For this review, take the finished solid that the model builds, in its own axes (mm). A direction names the side the tool comes from. Give positions to 0.01 mm unless a question says otherwise; leave off trailing zeros. Write each loop counter-clockwise with the first axis right and the second up, starting at its lowest first coordinate (ties: lowest second). Pieces come first, ordered by that corner, then holes. Notation, with made-up numbers: M 26,-33 L 36,-33 A18 ccw 36,-7 Z; hole C -3,73.25 d4. An arc over 180 degrees is marked long. Use one line per item in the form item = value. Start each with the question number.
Q1. Consider section B-B on x = 0. Write out the cut boundary in (y, z) (3 decimals), and give its area (3 significant figures).
Q2. Consider section D-D on x = -26. Write out the cut boundary in (y, z).
Q3. Clearance check with flat-ended pins moving along their axes: pin 1 Ø10 at (y, z) = (49.5, 45.5) entering from +X; pin 2 Ø10 at (y, z) = (11.5, -6) entering from +X; pin 3 Ø6 at (y, z) = (29.5, -36.5) entering from -X; pin 4 Ø1.6 at (x, z) = (-13.75, -5.41) entering from -Y. State where each tip first meets the part, or that it passes through.
Q4. Consider section A-A on y = 17. Write out the cut boundary in (x, z), and give its area (3 significant figures).
Q5. Consider section C-C on z = 0. Write out the cut boundary in (x, y) (3 decimals), and give its area (3 significant figures).
Q6. For probe 1 along Z at (x, y) = (0, 27); probe 2 along Z at (x, y) = (34, 36); probe 3 along X at (y, z) = (9, -13), list the stretches that pass through material, from the lowest coordinate up. Write a range as [from, to].
Q7. Mouldability with a two-part tool opening along Z and no side actions: class faces 1 (the cylindrical face through (41.569, 27.608, 17.235)), 2 (the cylindrical face through (26.34, 29.64, -41.32)) as released by +Z, released by -Z, zero draft, split by the parting line, or undercut.
Q8. Tool access review of faces 3 (the flat face through (38, 38, -1)), 4 (the flat face through (-15, 5, 0)), 5 (the flat face through (-26.9, 2.03, -20.31)): name each direction out of +Z, -Z, +X, -X, +Y, -Y from which nothing blocks a thin tool from reaching the whole face with its end or side.
```python
from build123d import *

# Parameters (mm, degrees)
SALIENTE_EXTRUIR2_DEPTH = 4
CROQUIS4_W              = 8
CROQUIS4_H              = 26
SALIENTE_EXTRUIR4_DEPTH = 34
CORTAR_EXTRUIR1_REACH   = 35.75
CROQUIS5_W              = 10
CROQUIS5_H              = 24
CROQUIS6_R              = 1.3
CORTAR_EXTRUIR2_DEPTH   = 7
SALIENTE_EXTRUIR5_DEPTH = 38
CROQUIS10_R             = 49
CROQUIS10_R_2           = 45
SALIENTE_EXTRUIR6_DEPTH = 56
CORTAR_EXTRUIR3_DEPTH   = 38
CROQUIS12_R             = 60.625
CROQUIS12_R_2           = 49
SALIENTE_EXTRUIR8_DEPTH = 4
CROQUIS13_R             = 3.1645
CORTAR_EXTRUIR5_DEPTH   = 14
CROQUIS14_R             = 1.3
CORTAR_EXTRUIR6_DEPTH   = 5
REDONDEO1_R             = 1


with BuildPart() as part:
    # Croquis1 → Saliente-Extruir2 (new body)
    with BuildSketch(Plane(origin=(0, 0, 0), x_dir=(1, 0, 0), z_dir=(0, 1, 0))):
        with BuildLine():
            Line((-11.25, 13.407227917), (-11.25, -12.592772083))
            Line((-11.25, -12.592772083), (-29.32452611, -34.133153509))
            ThreePointArc((-29.32452611, -34.133153509), (-44.999238647, 0.261765488), (-28.925442436, 34.47199994))
            Line((-28.925442436, 34.47199994), (-11.25, 13.407227917))
        make_face()
    extrude(amount=SALIENTE_EXTRUIR2_DEPTH)

    # Croquis4 → Saliente-Extruir4 (add)
    with BuildSketch(Plane(origin=(0, 4, 0), x_dir=(1, 0, 0), z_dir=(0, 1, 0))):
        with Locations((-15.25, 0.407227917)):
            Rectangle(CROQUIS4_W, CROQUIS4_H)
    extrude(amount=SALIENTE_EXTRUIR4_DEPTH)

    # Croquis5 → Cortar-Extruir1 (cut, up to next)
    with BuildSketch(Plane(origin=(-11.25, 0, 0), x_dir=(0, 0, -1), z_dir=(1, 0, 0)), mode=Mode.PRIVATE) as cortar_extruir1_sk1:
        with Locations((0.407227917, 17)):
            Rectangle(CROQUIS5_W, CROQUIS5_H)
    cortar_extruir1_tool1 = extrude(cortar_extruir1_sk1.sketch, amount=-CORTAR_EXTRUIR1_REACH, mode=Mode.PRIVATE) & part.part
    add(cortar_extruir1_tool1.solids().sort_by_distance((-11.25, 17, -0.407228))[0], mode=Mode.SUBTRACT)

    # Croquis6 → Cortar-Extruir2 (cut)
    with BuildSketch(Plane(origin=(0, 38, 0), x_dir=(1, 0, 0), z_dir=(0, 1, 0))):
        with Locations((-13.75, 5.407227917)):
            Circle(CROQUIS6_R)
        with Locations((-14.009261416, -4.592772083)):
            Circle(CROQUIS6_R)
    extrude(amount=-CORTAR_EXTRUIR2_DEPTH, mode=Mode.SUBTRACT)



with BuildPart() as body_2:
    # Croquis8 → Saliente-Extruir5 (new body)
    with BuildSketch(Plane(origin=(0, 0, 0), x_dir=(1, 0, 0), z_dir=(0, 1, 0))):
        with BuildLine():
            Line((31.75, 13.407227917), (31.75, -12.617796762))
            Line((31.75, -12.617796762), (43.287959819, -12.617796762))
            ThreePointArc((43.287959819, -12.617796762), (45.08754045, 0.412257936), (43.05, 13.407227917))
            Line((43.05, 13.407227917), (31.75, 13.407227917))
        make_face()
    extrude(amount=SALIENTE_EXTRUIR5_DEPTH)


with BuildPart() as part_1:
    add(part.part)

    add(body_2.part)  # Saliente-Extruir6 merges body 2
    # Croquis10 → Saliente-Extruir6 (add)
    with BuildSketch(Plane(origin=(0, 0, 0), x_dir=(1, 0, 0), z_dir=(0, 1, 0))):
        Circle(CROQUIS10_R)
        Circle(CROQUIS10_R_2, mode=Mode.SUBTRACT)
    extrude(amount=SALIENTE_EXTRUIR6_DEPTH)

    # Croquis11 → Cortar-Extruir3 (cut)
    with BuildSketch(Plane(origin=(0, 4, 0), x_dir=(1, 0, 0), z_dir=(0, 1, 0))):
        with BuildLine():
            Line((-24.25, 17.136853161), (-24.25, -15.043146839))
            Line((-24.25, -15.043146839), (-29.477670597, -21.308692316))
            ThreePointArc((-29.477670597, -21.308692316), (-38.734718404, 1.046853161), (-29.477670597, 23.402398638))
            Line((-29.477670597, 23.402398638), (-24.25, 17.136853161))
        make_face()
    extrude(amount=-CORTAR_EXTRUIR3_DEPTH, mode=Mode.SUBTRACT)

    # Croquis12 → Saliente-Extruir8 (add)
    with BuildSketch(Plane(origin=(0, 0, 0), x_dir=(1, 0, 0), z_dir=(0, 1, 0))):
        Circle(CROQUIS12_R)
        Circle(CROQUIS12_R_2, mode=Mode.SUBTRACT)
    extrude(amount=SALIENTE_EXTRUIR8_DEPTH)

    # Croquis13 → Cortar-Extruir5 (cut)
    with BuildSketch(Plane(origin=(0, 0, 0), x_dir=(1, 0, 0), z_dir=(0, 1, 0))):
        with Locations((-39.815475686, 37.946645437)):
            Circle(CROQUIS13_R)
        with Locations((37.944524314, 39.81473439)):
            Circle(CROQUIS13_R)
        with Locations((39.814027902, -37.94526561)):
            Circle(CROQUIS13_R)
        with Locations((-37.945972098, -39.813354563)):
            Circle(CROQUIS13_R)
    extrude(amount=CORTAR_EXTRUIR5_DEPTH, mode=Mode.SUBTRACT)

    # Croquis14 → Cortar-Extruir6 (cut)
    with BuildSketch(Plane(origin=(0, 38, 0), x_dir=(1, 0, 0), z_dir=(0, 1, 0))):
        with Locations((34.25, 5.407227917)):
            Circle(CROQUIS14_R)
        with Locations((34.25, -4.617796762)):
            Circle(CROQUIS14_R)
    extrude(amount=-CORTAR_EXTRUIR6_DEPTH, mode=Mode.SUBTRACT)

    # Redondeo1
    redondeo1_edges = [part_1.edges().sort_by_distance(p)[0] for p in [
        (-41.110472098, 4, 39.813354563),
        (36.649527902, 4, 37.94526561),
        (34.780024314, 4, -39.81473439),
        (-42.979975686, 4, -37.946645437),
    ]]
    fillet(redondeo1_edges, radius=REDONDEO1_R)


solid = part_1.part
```
Working result:
q1.outline = M 0,-60.625 L 4,-60.625 L 4,-49 L 56,-49 L 56,-45 L 0,-45 Z; M 0,45 L 56,45 L 56,49 L 4,49 L 4,60.625 L 0,60.625 Z
q1.area = 541 mm²
q2.outline = M 0,-54.77 L 4,-54.77 L 4,-41.53 L 56,-41.53 L 56,-36.73 L 0,-36.73 Z; M 0,-30.99 L 4,-30.99 L 4,-19.23 L 0,-19.23 Z; M 0,17.14 L 4,17.14 L 4,30.17 L 0,30.17 Z; M 0,36.73 L 56,36.73 L 56,41.53 L 4,41.53 L 4,54.77 L 0,54.77 Z
q3.pin_1 = 27.58
q3.pin_2 = 48.99
q3.pin_3 = -35.76
q3.pin_4 = 0
q4.outline = C 0,0 d98; M -19.25,-13.41 L -11.25,-13.41 L -11.25,-5.41 L -19.25,-5.41 Z; M -19.25,4.59 L -11.25,4.59 L -11.25,12.59 L -19.25,12.59 Z; hole M 31.75,-13.41 L 31.75,12.62 L 43.19,12.62 A45 ccw long 42.96,-13.41 Z
q4.area = 1,640 mm²
q5.outline = M -60.625,0 L -38.717,0 L -38.717,4 L -45,4 L -45,56 L -49,56 L -49,4 L -60.625,4 Z; M -24.25,0 L -11.25,0 L -11.25,5 L -19.25,5 L -19.25,4 L -24.25,4 Z; M -19.25,29 L -11.25,29 L -11.25,38 L -19.25,38 Z; M 31.75,0 L 60.625,0 L 60.625,4 L 49,4 L 49,56 L 45,56 L 45,38 L 31.75,38 Z
q5.area = 1,200 mm²
q6.probe_1 = [-49, -45], [45, 49]
q6.probe_2 = [-35.28, -29.48], [-13.41, -6.68], [-4.13, 3.34], [5.89, 12.62], [29.48, 35.28]
q6.probe_3 = [-47.24, -43.08], [-19.25, -11.25], [31.75, 47.24]
q7.face_1 = undercut
q7.face_2 = split by the parting line
q8.face_3 = +Y
q8.face_4 = none
q8.face_5 = +Y, -Y
